```python
from build123d import *

# Parameters (mm, degrees)
F1_DEPTH   = 11.938
F2_DEPTH   = 9.652
F3_SIZE2   = 2.54
F3_SIZE    = 7.62
F3_2_SIZE2 = 2.54
F3_2_SIZE  = 7.62
F3_3_SIZE2 = 2.54
F3_3_SIZE  = 7.62
F4_SIZE2   = 7.62
F4_SIZE    = 2.54
F5_R       = 2.53999
F6_R       = 3.0383713325
F7_DEPTH   = 25.4


# Not quite as in the source:
# - a fillet or chamfer is up to 0.001 mm smaller than in the source, because OpenCascade refuses the exact size


with BuildPart() as f1:
    # F0 (on Front) → F1 (new body)
    with BuildSketch(Plane.XZ):
        Polygon((-6.8888153673, -10.4809178157), (-4.5539487758, -8.1460512242), (8.1460512242, 4.5539487758), (10.4809178157, 6.8888153673), (6.8888153673, 10.4809178157), (4.5539487758, 8.1460512242), (-8.1460512242, -4.5539487758), (-10.4809178157, -6.8888153673), align=None)
    extrude(amount=F1_DEPTH)

    # F0 (on Front) → F2 (join)
    with BuildSketch(Plane.XZ):
        Polygon((-8.1460512242, 37.6100512242), (-8.1460512242, -4.5539487758), (4.5539487758, 8.1460512242), (4.5539487758, 37.6100512242), (0, 37.6100512242), align=None)
        Polygon((8.1460512242, 4.5539487758), (-4.5539487758, -8.1460512242), (37.6100512242, -8.1460512242), (37.6100512242, 0), (37.6100512242, 4.5539487758), align=None)
    extrude(amount=F2_DEPTH)

    # F3
    f3_edges = [f1.edges().sort_by_distance(p)[0] for p in [
        (-8.146051, -4.826, 37.610051),
    ]]
    f3_side = f1.faces().sort_by_distance((-8.146051, -4.826, 16.528051))[0]
    chamfer(f3_edges, length=F3_SIZE, length2=F3_SIZE2, reference=f3_side)

    # F3#2
    f3_2_edges = [f1.edges().sort_by_distance(p)[0] for p in [
        (4.553949, -4.826, 37.610051),
    ]]
    f3_2_side = f1.faces().sort_by_distance((4.553949, -4.826, 22.878051))[0]
    chamfer(f3_2_edges, length=F3_2_SIZE, length2=F3_2_SIZE2, reference=f3_2_side)

    # F3#3
    f3_3_edges = [f1.edges().sort_by_distance(p)[0] for p in [
        (37.610051, -4.826, 4.553949),
    ]]
    f3_3_side = f1.faces().sort_by_distance((22.878051, -4.826, 4.553949))[0]
    chamfer(f3_3_edges, length=F3_3_SIZE, length2=F3_3_SIZE2, reference=f3_3_side)

    # F4
    f4_edges = [f1.edges().sort_by_distance(p)[0] for p in [
        (37.610051, -4.826, -8.146051),
    ]]
    f4_side = f1.faces().sort_by_distance((37.610051, -4.826, -3.066051))[0]
    chamfer(f4_edges, length=F4_SIZE, length2=F4_SIZE2, reference=f4_side)

    # F5 (radius 2.54 in the source; OpenCascade refuses exactly that, so slightly less here)
    f5_edges = [f1.edges().sort_by_distance(p)[0] for p in [
        (-10.480918, -5.969, -6.888815),
        (-6.888815, -5.969, -10.480918),
    ]]
    fillet(f5_edges, radius=F5_R)

    # F6 (on face) → F7 (cut)
    with BuildSketch(Plane.XZ.offset(11.938)):
        with Locations((9.8638704833, 9.8638704833)):
            Circle(F6_R)
    extrude(amount=-F7_DEPTH, mode=Mode.SUBTRACT)


solid = f1.part
```
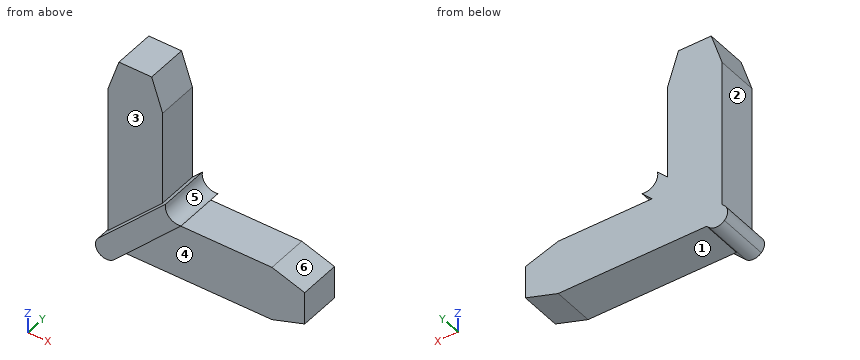
Verification items for the finished model (mm, model axes). Face numbers are marked on the shaded views. A direction names the side the tool comes from. Coordinates: 2 decimals unless noted, no trailing zeros. Write each loop counter-clockwise with the first axis right and the second up, starting at its lowest first coordinate (ties: lowest second). Pieces come first, ordered by that corner, then holes. Notation, with made-up numbers: (64.25, 87) - (106.25, 87) arc R4 cw to (106.25, 94) - close; hole circle Ø9 at (15, 58). An arc over 180 degrees is marked (long way). Write item = value, one per line.
Q1. Material ranges on L1, parallel to X at y = -0.25, z = 29; L2, parallel to Y at x = 20.5, z = 2, recorded low to high. Write a range as from..to.
Answer:
L1 = -8.15..4.55
L2 = -9.65..0
Q2. Access from +Z, -Z, +X, -X, +Y, -Y to the whole of each face (thin tool, end or side, straight path). Record for the marked faces 1, 2 and 3.
Answer:
face_1 = -Z, +X, +Y, -Y
face_2 = +Z, -X, +Y, -Y
face_3 = +Z, -X, -Y
Q3. Mould release check, pull along Z, two halves, no side actions. Record for the marked faces 4, 5 and 6: released by +Z, released by -Z, zero draft, split by the parting line, or undercut.
Answer:
face_4 = zero draft
face_5 = undercut
face_6 = released by +Z
Q4. Go/stop test with flat-tipped pins: pin 1 Ø1.5 at (y, z) = (-3.5, 31.5) entering from -X; pin 2 Ø14 at (x, z) = (19, 1) entering from -Y; pin 3 Ø3 at (y, z) = (-6, 5.5) entering from -X; pin 4 Ø8 at (x, z) = (9, 18) entering from -Y. Record where each tip stops, or that it passes through.
Answer:
pin_1 = -7.89
pin_2 = -9.65
pin_3 = -8.15
pin_4 = through
Q5. Cross-section at B-B (x = -0.5). Enter the section's corners in (y, z).
Answer:
outline = (-11.94, -4.09) - (-9.65, -4.09) - (-9.65, -8.15) - (0, -8.15) - (0, 37.61) - (-9.65, 37.61) - (-9.65, 3.09) - (-11.94, 3.09) - close
Q6. Cross-section at C-C (z = 25.5). Enter the section's corners in (x, y).
Answer:
outline = (-8.15, -9.65) - (4.55, -9.65) - (4.55, 0) - (-8.15, 0) - close
